```python
from build123d import *

# Parameters (mm, degrees)
F0_W     = 24
F0_H     = 16
F1_DEPTH = 48
F2_W     = 48
F2_H     = 24
F3_DEPTH = 31.991146
F4_W     = 48
F4_H     = 24
F5_DEPTH = 8


with BuildPart() as f1:
    # F0 (on Front) → F1 (new body)
    with BuildSketch(Plane.XZ):
        Polygon((-49.863074, 31.991146), (-50.615804, 0), (57.384196, 0), (57.384196, 56), (45.384196, 56), (45.384196, 64), (21.384196, 64), (21.384196, 56), (9.384196, 56), (9.384196, 31.991146), align=None)
        with Locations((33.384196, 40)):
            Rectangle(F0_W, F0_H, mode=Mode.SUBTRACT)
    extrude(amount=F1_DEPTH)

    # F2 (on Top) → F3 (cut, through all)
    with BuildSketch(Plane.XY):
        with Locations((-14.853436, -22.356194)):
            Rectangle(F2_W, F2_H)
    extrude(amount=F3_DEPTH, mode=Mode.SUBTRACT)

    # F4 (on Top) → F5 (join)
    with BuildSketch(Plane.XY):
        with Locations((-14.719842, -22.231252)):
            Rectangle(F4_W, F4_H)
    extrude(amount=F5_DEPTH)


solid = f1.part
```
Model file for the job. Use its own axes, mm. A direction names the side the tool comes from. Coordinates: 2 decimals unless noted, no trailing zeros. Write each loop counter-clockwise with the first axis right and the second up, starting at its lowest first coordinate (ties: lowest second). Pieces come first, ordered by that corner, then holes. Notation, with made-up numbers: (64.25, 36) - (68.25, 36) arc R31 cw to (68.25, 69) - close; hole circle Ø3 at (-17, -6). An arc over 180 degrees is marked (long way). One line per question, with ' | ' between items. Start each with the question number.
Q1. Pin check, flat tips, straight feed: pin 1 (9.5 mm diameter, centred on x = -26.5, z = 23.5, fed in from +Y); pin 2 (3.5 mm diameter, centred on x = 15, y = -14, fed in from +Z); pin 3 (6 mm diameter, centred on x = -8.5, y = -41, fed in from +Z); pin 4 (8 mm diameter, centred on y = -31.5, z = 8.5, fed in from -X). Stop position of each tip, or through.
Q2. 3-axis set-ups, long thin cutter, end or side, ignore diameter. For faces 4 (the face through (45.384, -24, 60)), 5 (the face through (15, -24, 56)), 6 (the face through (45.384, -24, 40)), 7 (the face through (9.147, -23, 19)): which of +Z, -Z, +X, -X, +Y, -Y reach the whole face in a straight line?
Q3. Cut at C-C, the plane z = 43.5. List the corners of the cut face in (x, y), then the cut area to 3 significant figures.
Q4. Cut at A-A, the plane y = -28.5. List the corners of the cut face in (x, z), then the cut area to 3 significant figures.
Q5. Pull direction Y, two halves, no side cores. Call faces 1 (the face through (51, -24, 56)), 2 (the face through (15, 0, 25)), 3 (the face through (-15, -34.356, 16)): pulls with the +Y half, pulls with the -Y half, needs draft (parallel to the pull), parting line crosses it, or undercut.
Q6. Drill centre lines: line 1 (X direction, y = -33.5, z = 38); line 2 (Z direction, x = 25, y = -4.5); line 3 (Y direction, x = -17, z = 24.5). Where is each one in solid material? Low to high. Write a range as [from, to].
Q7. Cut at D-D, the plane y = -44. List the corners of the cut face in (x, z), then the cut area to 3 significant figures.
Q8. Cut at B-B, the plane x = 35.5. List the corners of the cut face in (y, z), then the cut area to 3 significant figures.
Answer below:
1) pin 1: y = 0 | pin 2: z = 56 | pin 3: z = 31.99 | pin 4: x = -50.51
2) face 4: +Z, +X, +Y, -Y | face 5: +Z, -X, +Y, -Y | face 6: +Y, -Y | face 7: +Z
3) outline: (9.38, -48) - (21.38, -48) - (21.38, 0) - (9.38, 0) - close; (45.38, -48) - (57.38, -48) - (57.38, 0) - (45.38, 0) - close | area: 1,150 mm^2
4) outline: (-50.62, 0) - (-38.85, 0) - (-38.85, 31.99) - (-49.86, 31.99) - close; (-38.72, 0) - (57.38, 0) - (57.38, 56) - (45.38, 56) - (45.38, 64) - (21.38, 64) - (21.38, 56) - (9.38, 56) - (9.38, 31.99) - (9.15, 31.99) - (9.15, 8) - (-38.72, 8) - close; hole (21.38, 32) - (45.38, 32) - (45.38, 48) - (21.38, 48) - close | area: 3,250 mm^2
5) face 1: needs draft | face 2: pulls with the +Y half | face 3: undercut
6) line 1: [9.38, 21.38], [45.38, 57.38] | line 2: [0, 32], [48, 64] | line 3: [-48, -34.36], [-10.36, 0]
7) outline: (-50.62, 0) - (57.38, 0) - (57.38, 56) - (45.38, 56) - (45.38, 64) - (21.38, 64) - (21.38, 56) - (9.38, 56) - (9.38, 31.99) - (-49.86, 31.99) - close; hole (21.38, 32) - (45.38, 32) - (45.38, 48) - (21.38, 48) - close | area: 4,400 mm^2
8) outline: (-48, 0) - (0, 0) - (0, 32) - (-48, 32) - close; (-48, 48) - (0, 48) - (0, 64) - (-48, 64) - close | area: 2,300 mm^2
